```python
from build123d import *

# Parameters (mm, degrees)
SKETCH1_W           = 202.8
SKETCH1_H           = 28
SKETCH1_R           = 2.125
BOSS_EXTRUDE1_DEPTH = 3.175
FILLET1_R           = 2


with BuildPart() as part:
    # Sketch1 → Boss-Extrude1 (new body)
    with BuildSketch(Plane.XY):
        Rectangle(SKETCH1_W, SKETCH1_H)
        with Locations((85.05, 6)):
            Circle(SKETCH1_R, mode=Mode.SUBTRACT)
        with Locations(Location((85.05, -6, 0), (0, 0, 180))):
            Circle(SKETCH1_R, mode=Mode.SUBTRACT)
        with Locations((-85.05, -6)):
            Circle(SKETCH1_R, mode=Mode.SUBTRACT)
        with Locations(Location((-85.05, 6, 0), (0, 0, 180))):
            Circle(SKETCH1_R, mode=Mode.SUBTRACT)
        with Locations((-35.05, 6)):
            Circle(SKETCH1_R, mode=Mode.SUBTRACT)
        with Locations(Location((-35.05, -6, 0), (0, 0, 180))):
            Circle(SKETCH1_R, mode=Mode.SUBTRACT)
        with Locations((35.05, -6)):
            Circle(SKETCH1_R, mode=Mode.SUBTRACT)
        with Locations(Location((35.05, 6, 0), (0, 0, 180))):
            Circle(SKETCH1_R, mode=Mode.SUBTRACT)
    extrude(amount=BOSS_EXTRUDE1_DEPTH)

    # Fillet1
    fillet1_edges = [part.edges().sort_by_distance(p)[0] for p in [
        (101.4, -14, 1.5875),
        (-101.4, -14, 1.5875),
        (-101.4, 14, 1.5875),
        (101.4, 14, 1.5875),
    ]]
    fillet(fillet1_edges, radius=FILLET1_R)


solid = part.part
```
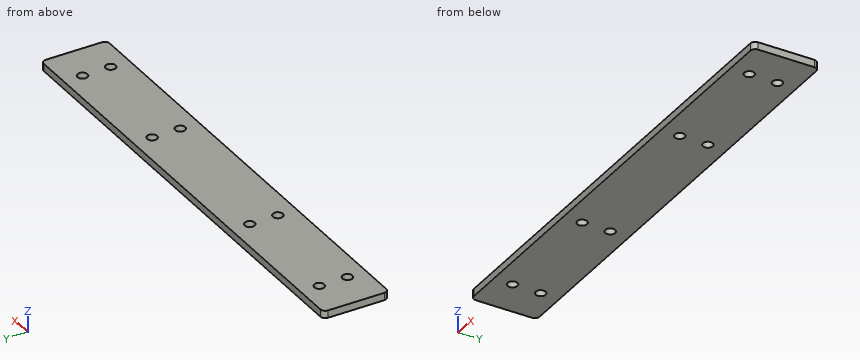
Design review of the part built by this model. Coordinates are the model's own, in mm. Round coordinates to 2 decimals unless told otherwise and drop trailing zeros. Write each loop counter-clockwise with the first axis right and the second up, starting at its lowest first coordinate (ties: lowest second). Pieces come first, ordered by that corner, then holes.
Item 1: We need section B-B on y = -6. Write out the cut boundary in (x, z) (3 decimals), and give its area (3 significant figures).
Item 2: For probe 1 along Y at (x, z) = (35.05, 1.9) (3 decimals); probe 2 along X at (y, z) = (5, 0.3) (3 decimals); probe 3 along X at (y, z) = (-4.25, 2.15), list the stretches that pass through material, from the lowest coordinate up.
Item 3: We need section A-A on x = -85.05. Write out the cut boundary in (y, z) (3 decimals).
Item 4: We need section C-C on z = 0.65. State how many separate pieces and enclosed holes the cut face has, and give its area (3 significant figures).
Item 5: Clearance check with a flat-ended pin moving along its axis: pin 1 Ø7 at (x, y) = (35.05, 6) entering from -Z. State where the tip first meets the part, or that it passes through.
Returned:
1. outline: (-101.4, 0) - (-87.175, 0) - (-87.175, 3.175) - (-101.4, 3.175) - close; (-82.925, 0) - (-37.175, 0) - (-37.175, 3.175) - (-82.925, 3.175) - close; (-32.925, 0) - (32.925, 0) - (32.925, 3.175) - (-32.925, 3.175) - close; (37.175, 0) - (82.925, 0) - (82.925, 3.175) - (37.175, 3.175) - close; (87.175, 0) - (101.4, 0) - (101.4, 3.175) - (87.175, 3.175) - close
1. area: 590 mm2
2. probe 1: y = -14 to -8.125, -3.875 to 3.875, 8.125 to 14
2. probe 2: x = -101.4 to -86.925, -83.175 to -36.925, -33.175 to 33.175, 36.925 to 83.175, 86.925 to 101.4
2. probe 3: x = -101.4 to -86.26, -83.84 to -36.26, -33.84 to 33.84, 36.26 to 83.84, 86.26 to 101.4
3. outline: (-14, 0) - (-8.125, 0) - (-8.125, 3.175) - (-14, 3.175) - close; (-3.875, 0) - (3.875, 0) - (3.875, 3.175) - (-3.875, 3.175) - close; (8.125, 0) - (14, 0) - (14, 3.175) - (8.125, 3.175) - close
4. separate pieces: 1
4. enclosed holes: 8
4. area: 5,560 mm2
5. pin 1: stops at z = 0
